from build123d import *

# Parameters (mm, degrees)
SKETCH2_W                  = 25.4
SKETCH2_H                  = 12.7
BOSS_EXTRUDE1_DEPTH        = 6.35
SKETCH3_R                  = 0.5461
CUT_EXTRUDE1_DEPTH         = 7.35
SKETCH4_W                  = 50.8
SKETCH4_H                  = 12.7
BOSS_EXTRUDE2_DEPTH        = 6.35
F_8_0_199_DIAMETER_HOLE1_D = 2.54
F_6_32_TAPPED_HOLE3_D      = 2.7051
FILLET1_R                  = 1
SKETCH17_W                 = 12.7
SKETCH17_H                 = 12.7
BOSS_EXTRUDE3_DEPTH        = 2.54
F_6_32_TAPPED_HOLE4_D      = 2.7051
F_6_32_TAPPED_HOLE4_DEPTH  = 5.4864
F_6_32_TAPPED_HOLE4_TIP    = 0.81269403


with BuildPart() as part:
    # Sketch2 → Boss-Extrude1 (new body)
    with BuildSketch(Plane(origin=(0, 0, 0), x_dir=(1, 0, 0), z_dir=(0, 1, 0))):
        with Locations((12.7, -6.35)):
            Rectangle(SKETCH2_W, SKETCH2_H)
    extrude(amount=BOSS_EXTRUDE1_DEPTH)

    # Sketch3 → Cut-Extrude1 (cut, through all)
    with BuildSketch(Plane.XZ):
        with Locations((5.334, 9.1186)):
            Circle(SKETCH3_R)
        with Locations((5.334, 3.5814)):
            Circle(SKETCH3_R)
        with Locations((21.209, 3.5814)):
            Circle(SKETCH3_R)
        with Locations((21.209, 9.1186)):
            Circle(SKETCH3_R)
    extrude(amount=-CUT_EXTRUDE1_DEPTH, mode=Mode.SUBTRACT)

    # Sketch4 → Boss-Extrude2 (add)
    with BuildSketch(Plane(origin=(0, 6.35, 0), x_dir=(1, 0, 0), z_dir=(0, 1, 0))):
        with Locations((25.4, -6.35)):
            Rectangle(SKETCH4_W, SKETCH4_H)
    extrude(amount=BOSS_EXTRUDE2_DEPTH)

    # #8 (0.199) Diameter Hole1 (through all)
    with Locations(Plane(origin=(0, 0, 0), x_dir=(-1, 0, 0), z_dir=(0, -1, 0))):
        with Locations((-5.334, -3.5814), (-21.209, -3.5814), (-21.209, -9.1186), (-5.334, -9.1186)):
            Hole(F_8_0_199_DIAMETER_HOLE1_D / 2)

    # #6-32 Tapped Hole3 (through all)
    with Locations(Plane(origin=(0, 6.35, 0), x_dir=(-1, 0, 0), z_dir=(0, -1, 0))):
        with Locations((-33.02, -6.35), (-45.72, -6.35)):
            Hole(F_6_32_TAPPED_HOLE3_D / 2)

    # Fillet1
    fillet1_edges = [part.edges().sort_by_distance(p)[0] for p in [
        (50.8, 6.35, 6.35),
    ]]
    fillet(fillet1_edges, radius=FILLET1_R)

    # Sketch17 → Boss-Extrude3 (add)
    with BuildSketch(Plane.ZY):
        with Locations((6.35, 6.35)):
            Rectangle(SKETCH17_W, SKETCH17_H)
    extrude(amount=BOSS_EXTRUDE3_DEPTH)

    # #6-32 Tapped Hole4
    with Locations(Plane.ZY.offset(2.54)):
        with Locations((6.35, 6.35)):
            Hole(F_6_32_TAPPED_HOLE4_D / 2, depth=F_6_32_TAPPED_HOLE4_DEPTH)
            with Locations((0, 0, -(F_6_32_TAPPED_HOLE4_DEPTH + F_6_32_TAPPED_HOLE4_TIP / 2))):  # 118° drill point
                Cone(0, F_6_32_TAPPED_HOLE4_D / 2, F_6_32_TAPPED_HOLE4_TIP, mode=Mode.SUBTRACT)


solid = part.part
Read the model definition and answer for the solid it produces. Units are mm, in the model's axes. A direction names the side the tool comes from. Coordinates: 2 decimals unless noted, no trailing zeros. Order: outer loops, then holes, each group sorted by start corner. A loop starts at its lowest first (then second) coordinate and runs counter-clockwise, first axis right, second up. Notation, with made-up numbers: M 73,24 L 127,24 A8 cw 127,39 Z; hole C 50,7.25 d9. An arc over 180 degrees is marked long. Put each result on its own line as item: value. Start each with the question number.
Item 1: Consider probe 1 along X at (y, z) = (11.75, 6.35); probe 2 along Z at (x, y) = (5.5, 10); probe 3 along Z at (x, y) = (4.5, 3.75). Determine where each line is inside the solid, lowest interval first. Write a range as [from, to].
Item 2: Section D-D, the plane y = 2 is taken. Determine the outline of the cut face in (x, z).
Item 3: Given pin 1 Ø4.5 at (x, z) = (33.02, 6.35) entering from +Y; pin 2 Ø4 at (x, z) = (40.5, 8) entering from -Y; pin 3 Ø6 at (y, z) = (2.5, 1.5) entering from +X, each flat-ended and moving along its own axis, determine where each tip first touches the part or whether it passes through.
Item 4: Section C-C, the plane x = 45.72 is taken. Determine the outline of the cut face in (y, z), plus the area to 3 significant figures.
Item 5: Section B-B, the plane z = 12 is taken. Determine the outline of the cut face in (x, y).
Item 6: For faces 1 (the face through (0.2, 5.5, 7.4)), 2 (the face through (34.31, 9.57, 5.94)), 3 (the face through (25.4, 3, 6)), determine the directions among +Z, -Z, +X, -X, +Y, -Y from which every point of the face is accessible in a straight line to the end or side of a thin tool.
Item 7: Section A-A, the plane x = 6 is taken. Determine the outline of the cut face in (y, z).
Item 8: The mould has two halves that part along X. Classify faces 4 (the face through (5.06, 6.44, 10.36)), 5 (the face through (-2.54, 8, 6)), 6 (the face through (37, 6.35, 6)): +X half, -X half, draft (parallel to the pull), parting line (faces both ways), or undercut.
Computed:
1. probe 1: x = [-2.54, 31.67], [34.37, 44.37], [47.07, 50.8]
1. probe 2: z = [0, 2.32], [4.84, 7.86], [10.38, 12.7]
1. probe 3: z = [0, 2.62], [4.54, 8.16], [10.08, 12.7]
2. outline: M -2.54,0 L 25.4,0 L 25.4,12.7 L -2.54,12.7 Z; hole C 5.33,3.58 d2.54; hole C 5.33,9.12 d2.54; hole C 21.21,3.58 d2.54; hole C 21.21,9.12 d2.54
3. pin 1: stops at y = 12.7
3. pin 2: stops at y = 6.35
3. pin 3: stops at x = 25.4
4. outline: M 6.35,0 L 12.7,0 L 12.7,5 L 6.35,5 Z; M 6.35,7.7 L 12.7,7.7 L 12.7,12.7 L 6.35,12.7 Z
4. area: 63.5 mm2
5. outline: M -2.54,0 L 25.4,0 L 25.4,6.35 L 49.8,6.35 A1 ccw 50.8,7.35 L 50.8,12.7 L -2.54,12.7 Z
6. face 1: -X
6. face 2: +Y, -Y
6. face 3: +Z, -Z, +X, -Y
7. outline: M 0,0 L 12.7,0 L 12.7,2.5 L 0,2.5 Z; M 0,4.66 L 12.7,4.66 L 12.7,8.04 L 0,8.04 Z; M 0,10.2 L 12.7,10.2 L 12.7,12.7 L 0,12.7 Z
8. face 4: undercut
8. face 5: -X half
8. face 6: draft
